Could you check a few things on this drawing? It's one solid part, dimensions in mm from its lowest x, y, z. A direction names the side the tool comes from. Round coordinates to 2 decimals unless told otherwise and drop trailing zeros. Write each loop counter-clockwise with the first axis right and the second up, starting at its lowest first coordinate (ties: lowest second). Pieces come first, ordered by that corner, then holes. Notation, with made-up numbers: (82.25, 55) -> (108.25, 55) arc R27 cw to (108.25, 82) -> close; hole circle Ø11 at (46.5, 53). An arc over 180 degrees is marked (long way). Answer in a Markdown table with one row per item.
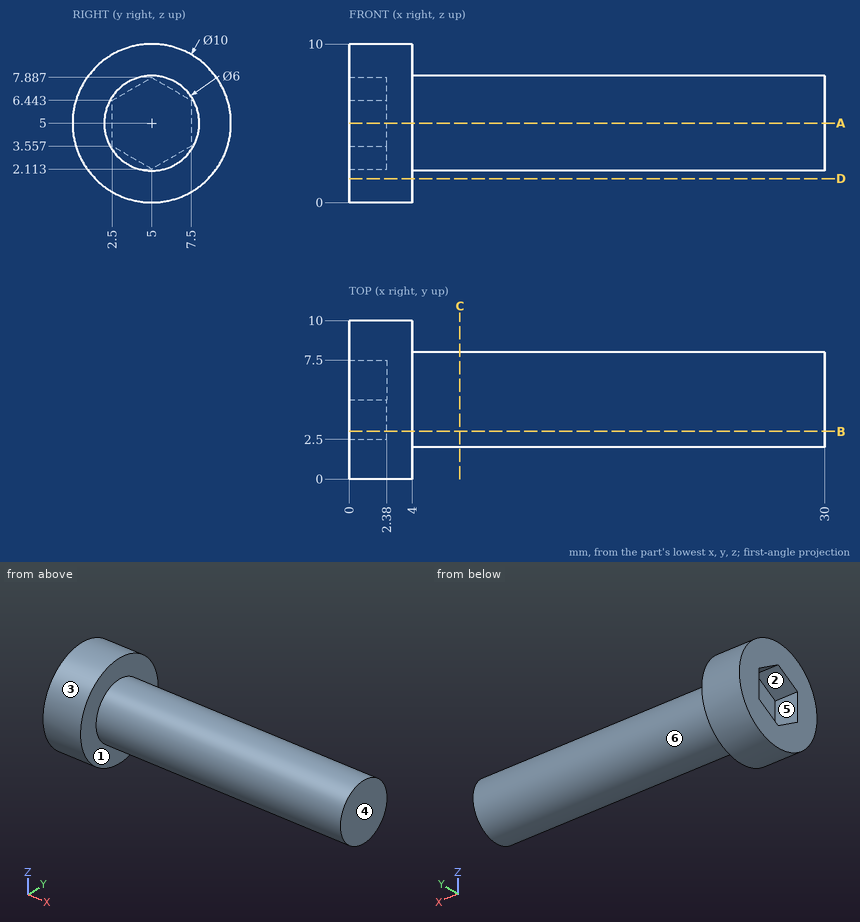
1) For the marked faces 4, 5 and 6, which set-ups out of +Z, -Z, +X, -X, +Y, -Y let a thin tool reach every point of the face, with its end or its side?
Findings:
| item | result |
|---|---|
| face 4 | +Z, -Z, +X, +Y, -Y |
| face 5 | -X |
| face 6 | +X |
2) Imagine slicing it at A-A, the plane z = 5. Please give me the cut outline in (x, y).
Findings:
| item | result |
|---|---|
| outline | (0, 0) -> (4, 0) -> (4, 2) -> (30, 2) -> (30, 8) -> (4, 8) -> (4, 10) -> (0, 10) -> (0, 7.5) -> (2.38, 7.5) -> (2.38, 2.5) -> (0, 2.5) -> close |
3) For pin 1 (2 mm diameter, centred on x = 15, y = 1.5, fed in from -Z); pin 2 (1.5 mm diameter, centred on x = 21, y = 7.5, fed in from +Z); pin 3 (1.5 mm diameter, centred on x = 15, z = 7, fed in from +Y), each with a flat end and sliding along its axis, tell me the tip position at first contact or that it passes through.
Findings:
| item | result |
|---|---|
| pin 1 | stops at z = 3.34 |
| pin 2 | stops at z = 7.44 |
| pin 3 | stops at y = 7.73 |
4) Please list where these lines run through material, in increasing order: line 1 (X direction, y = 6, z = 8.75); line 2 (X direction, y = 4.5, z = 4.5); line 3 (Y direction, x = 25, z = 5.75) (1 decimal).
Findings:
| item | result |
|---|---|
| line 1 | x = 0 to 4 |
| line 2 | x = 2.38 to 30 |
| line 3 | y = 2.1 to 7.9 |
5) Thinking about a two-plate mould opening in Y: for the marked faces 1, 2 and 3, which applies, +Y half, -Y half, draft (parallel to the pull), parting line (faces both ways), or undercut?
Findings:
| item | result |
|---|---|
| face 1 | draft |
| face 2 | undercut |
| face 3 | parting line |
6) Imagine slicing it at C-C, the plane x = 7. Please give me the cut outline in (y, z), plus the area to 3 significant figures.
Findings:
| item | result |
|---|---|
| outline | circle Ø6 at (5, 5) |
| area | 28.3 mm^2 |
7) Imagine slicing it at B-B, the plane y = 3. Please give me the cut outline in (x, z).
Findings:
| item | result |
|---|---|
| outline | (0, 0.42) -> (4, 0.42) -> (4, 2.76) -> (30, 2.76) -> (30, 7.24) -> (4, 7.24) -> (4, 9.58) -> (0, 9.58) -> (0, 6.73) -> (2.38, 6.73) -> (2.38, 3.27) -> (0, 3.27) -> close |
8) Imagine slicing it at D-D, the plane z = 1.5. Please give me the cut outline in (x, y).
Findings:
| item | result |
|---|---|
| outline | (0, 1.43) -> (4, 1.43) -> (4, 8.57) -> (0, 8.57) -> close |
